CAD build for the part. Positions are in the model's coordinates, mm. Face numbers are marked on the shaded views. A direction names the side the tool comes from. Give positions to 0.01 mm unless a question says otherwise; leave off trailing zeros. Loops run counter-clockwise (first coordinate to the right, second up) from the corner with the lowest first, then second, coordinate; pieces in that order, holes last.
```python
from build123d import *

# Parameters (mm, degrees)
PAD_DEPTH       = 2
SKETCH002_W     = 54.3
SKETCH002_H     = 22
PAD001_DEPTH    = 2
SKETCH003_R     = 2.95
PAD002_DEPTH    = 5
CHAMFER_SIZE    = 0.5
SKETCH004_W     = 6.85
SKETCH004_H     = 15
PAD003_DEPTH    = 20
SKETCH005_R     = 1.4
POCKET_DEPTH    = 15
SKETCH006_W     = 6.85
SKETCH006_H     = 15
PAD004_DEPTH    = 20
SKETCH007_R     = 1.4
POCKET001_DEPTH = 15
SKETCH008_W     = 54.3
SKETCH008_H     = 2
PAD005_DEPTH    = 38
SKETCH009_W     = 6.85
SKETCH009_H     = 15
PAD006_DEPTH    = 20
SKETCH010_R     = 1.4
POCKET002_DEPTH = 15
SKETCH011_W     = 6.85
SKETCH011_H     = 25.8
PAD007_DEPTH    = 20
SKETCH012_R     = 1.4
POCKET003_DEPTH = 15
SKETCH013_R     = 2.95
PAD008_DEPTH    = 5
CHAMFER001_SIZE = 0.5


with BuildPart() as body:
    # Sketch → Pad (new body)
    with BuildSketch(Plane.XY):
        Polygon((54.3, 19), (54.3, -19), (0, -19), (-18.1, -11), (-54.3, -11), (-54.3, 11), (-18.1, 11), (0, 19), align=None)
    extrude(amount=PAD_DEPTH)

    # Sketch002 (on Face2 of Pad) → Pad001 (join)
    with BuildSketch(Plane.XZ.offset(19)):
        with Locations((27.15, 11)):
            Rectangle(SKETCH002_W, SKETCH002_H)
    extrude(amount=PAD001_DEPTH)

    # Sketch003 (on Face10 of Pad001) → Pad002 (join)
    with BuildSketch(Plane.XZ.offset(21)):
        with Locations((37.25, 12)):
            Circle(SKETCH003_R)
    extrude(amount=PAD002_DEPTH)

    # Chamfer
    chamfer_edges = [body.edges().sort_by_distance(p)[0] for p in [
        (34.3, -26, 12),
    ]]
    chamfer(chamfer_edges, length=CHAMFER_SIZE)

    # Sketch004 (on Face18 of Chamfer) → Pad003 (join)
    with BuildSketch(Plane.XY.offset(2)):
        with Locations((3.425, -0.7)):
            Rectangle(SKETCH004_W, SKETCH004_H)
    extrude(amount=PAD003_DEPTH)

    # Sketch005 (on Face22 of Pad003) → Pocket (cut)
    with BuildSketch(Plane(origin=(0, 6.8, 0), x_dir=(-1, 0, 0), z_dir=(0, 1, 0))):
        with Locations((-3, 17)):
            Circle(SKETCH005_R)
        with Locations((-3, 7)):
            Circle(SKETCH005_R)
    extrude(amount=-POCKET_DEPTH, mode=Mode.SUBTRACT)

    # Sketch006 (on Face18 of Pocket) → Pad004 (join)
    with BuildSketch(Plane.XY.offset(2)):
        with Locations((50.875, -0.7)):
            Rectangle(SKETCH006_W, SKETCH006_H)
    extrude(amount=PAD004_DEPTH)

    # Sketch007 (on Face20 of Pad004) → Pocket001 (cut)
    with BuildSketch(Plane(origin=(0, 6.8, 0), x_dir=(-1, 0, 0), z_dir=(0, 1, 0))):
        with Locations((-51.3, 17)):
            Circle(SKETCH007_R)
        with Locations((-51.3, 7)):
            Circle(SKETCH007_R)
    extrude(amount=-POCKET001_DEPTH, mode=Mode.SUBTRACT)

    # Sketch008 (on Face18 of Pocket001) → Pad005 (join)
    with BuildSketch(Plane.XY.offset(2)):
        with Locations((-27.15, 10)):
            Rectangle(SKETCH008_W, SKETCH008_H)
    extrude(amount=PAD005_DEPTH)

    # Sketch009 (on Face25 of Pad005) → Pad006 (join)
    with BuildSketch(Plane.XZ.offset(-9)):
        with Locations((-50.875, 20.3)):
            Rectangle(SKETCH009_W, SKETCH009_H)
    extrude(amount=PAD006_DEPTH)

    # Sketch010 (on Face38 of Pad006) → Pocket002 (cut)
    with BuildSketch(Plane.XY.offset(27.8)):
        with Locations((-51.3, -6)):
            Circle(SKETCH010_R)
        with Locations((-51.3, 4)):
            Circle(SKETCH010_R)
    extrude(amount=-POCKET002_DEPTH, mode=Mode.SUBTRACT)

    # Sketch011 (on Face25 of Pocket002) → Pad007 (join)
    with BuildSketch(Plane.XZ.offset(-9)):
        with Locations((-3.425, 14.9)):
            Rectangle(SKETCH011_W, SKETCH011_H)
    extrude(amount=PAD007_DEPTH)

    # Sketch012 (on Face41 of Pad007) → Pocket003 (cut)
    with BuildSketch(Plane.XY.offset(27.8)):
        with Locations((-3, -6)):
            Circle(SKETCH012_R)
        with Locations((-3, 4)):
            Circle(SKETCH012_R)
    extrude(amount=-POCKET003_DEPTH, mode=Mode.SUBTRACT)

    # Sketch013 (on Face9 of Pocket003) → Pad008 (join)
    with BuildSketch(Plane(origin=(0, 0, 0), x_dir=(1, 0, 0), z_dir=(0, 0, -1))):
        with Locations((-37.25, -1)):
            Circle(SKETCH013_R)
    extrude(amount=PAD008_DEPTH)

    # Chamfer001
    chamfer001_edges = [body.edges().sort_by_distance(p)[0] for p in [
        (-40.2, 1, -5),
    ]]
    chamfer(chamfer001_edges, length=CHAMFER001_SIZE)


with BuildPart() as part_mirroring:
    # Part__Mirroring: instance of Body
    add(body.part.mirror(Plane(origin=(0, 0, 0), x_dir=(1, 0, 0), z_dir=(0, 1, 0))))


solid = part_mirroring.part
```
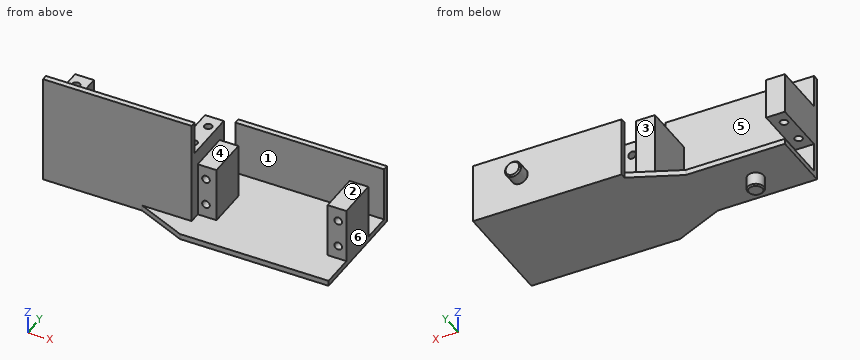
1. Saw through at B-B, the plane x = 3. List the corners of the cut face in (y, z), and give its area (3 significant figures).
Responses:
outline: (-19, 0) - (21, 0) - (21, 22) - (19, 22) - (19, 2) - (8.2, 2) - (8.2, 5.6) - (-6.8, 5.6) - (-6.8, 2) - (-19, 2) - close; (-6.8, 8.4) - (8.2, 8.4) - (8.2, 15.6) - (-6.8, 15.6) - close; (-6.8, 18.4) - (8.2, 18.4) - (8.2, 22) - (-6.8, 22) - close
area: 336 mm2
2. Probe line 1 along Y through (x, z) = (-3, 13.5); line 2 along Z through (x, y) = (3, 1); line 3 along X through (y, z) = (-4, 20). List the from-to ranges inside material, lowest first.
Responses:
line 1: y = -11 to -5.4, -2.6 to 4.6, 7.4 to 11
line 2: z = 0 to 5.6, 8.4 to 15.6, 18.4 to 22
line 3: x = -54.3 to -52.7, -49.9 to -47.45, -6.85 to -4.4, -1.6 to 6.85, 47.45 to 54.3
3. Tool access for the marked faces 1, 2 and 3: list every direction of +Z, -Z, +X, -X, +Y, -Y with a clear straight run to the whole face (end or side of a thin tool).
Responses:
face 1: +Z, +X, -X
face 2: +Z, +X, +Y, -Y
face 3: +Z, +X, -X, +Y
4. Drop flat-ended pins along their axis: pin 1 (3.5 mm diameter, centred on x = -49.5, y = 4, fed in from -Z); pin 2 (4 mm diameter, centred on y = 9, z = 27, fed in from +X); pin 3 (10 mm diameter, centred on x = 43, y = -6.5, fed in from +Z); pin 4 (1.5 mm diameter, centred on y = 13, z = 26.5, fed in from -X). Give the stop position or say it passes through.
Responses:
pin 1: stops at z = 0
pin 2: stops at x = 0
pin 3: stops at z = 22
pin 4: passes through
5. Saw through at A-A, the plane z = 17. Count the separate pieces of the cut face and the enclosed holes in it, and give its area (3 significant figures).
Responses:
separate pieces: 5
enclosed holes: 4
area: 588 mm2
6. Pull direction X, two halves, no side cores. Call the marked faces 4, 5 and 6: released by +X, released by -X, zero draft, split by the parting line, or undercut.
Responses:
face 4: zero draft
face 5: undercut
face 6: released by +X
7. Saw through at C-C, the plane y = 6. List the corners of the cut face in (x, z).
Responses:
outline: (-54.3, 0) - (54.3, 0) - (54.3, 22) - (47.45, 22) - (47.45, 2) - (6.85, 2) - (6.85, 22) - (0, 22) - (0, 27.8) - (-1.6, 27.8) - (-1.6, 12.8) - (-4.4, 12.8) - (-4.4, 27.8) - (-6.85, 27.8) - (-6.85, 2) - (-54.3, 2) - close; (-54.3, 12.8) - (-52.7, 12.8) - (-52.7, 27.8) - (-54.3, 27.8) - close; (-49.9, 12.8) - (-47.45, 12.8) - (-47.45, 27.8) - (-49.9, 27.8) - close; hole circle Ø2.8 at (3, 7); hole circle Ø2.8 at (3, 17); hole circle Ø2.8 at (51.3, 7); hole circle Ø2.8 at (51.3, 17)
8. Saw through at D-D, the plane z = 7. List the corners of the cut face in (x, y), and give its area (3 significant figures).
Responses:
outline: (-54.3, -11) - (0, -11) - (0, -6.8) - (1.6, -6.8) - (1.6, 8.2) - (0, 8.2) - (0, 11) - (-6.85, 11) - (-6.85, -9) - (-54.3, -9) - close; (0, 19) - (54.3, 19) - (54.3, 21) - (0, 21) - close; (4.4, -6.8) - (6.85, -6.8) - (6.85, 8.2) - (4.4, 8.2) - close; (47.45, -6.8) - (49.9, -6.8) - (49.9, 8.2) - (47.45, 8.2) - close; (52.7, -6.8) - (54.3, -6.8) - (54.3, 8.2) - (52.7, 8.2) - close
area: 476 mm2
